Autodesk Inventor part; units mm, degrees
ref_plane "YZ Plane" through (0, 0, 0) normal (1, 0, 0) x (0, 1, 0)
ref_plane "XZ Plane" through (0, 0, 0) normal (0, 1, 0) x (-1, 0, 0)
ref_plane "XY Plane" through (0, 0, 0) normal (0, 0, 1) x (1, 0, 0)
ref_plane "РабПлоскость1" through (0, 0, 0) normal (0, 0, 1) x (1, 0, 0)
sketch "Эскиз1" plane through (0, 0, 0) normal (0, 0, 1) x (1, 0, 0)
  circle A0 centre (-0.0013, 107.169) radius 13.15
  circle A1 centre (-0.0025, 107.6908) radius 11.9
  point P0 (0, 0)
extrude "Выдавливание1" add sketch "Эскиз1" against normal blind 10 contours A0 | A1
sketch "Эскиз2" plane through (-0.0013, 107.169, 0) normal (0, 0, 1) x (1, 0, 0)
  circle A0 centre (0, 0) radius 15.5
  point P0 (0.0013, -107.169)
  dimension "d2" = 31
extrude "Выдавливание2" add sketch "Эскиз2" along normal blind 5.2
sketch "Эскиз3" plane through (-0.0013, 107.169, 5.2) normal (0, 0, 1) x (1, 0, 0)
  circle A0 centre (0, 0) radius 11.9
  point P0 (0.0013, -107.169)
  dimension "d5" = 23.8
extrude "Выдавливание3" add sketch "Эскиз3" along normal blind 20
sketch "Эскиз4" plane through (-0.0013, 107.169, 25.2) normal (0, 0, 1) x (1, 0, 0)
  circle A0 centre (0, 0) radius 6.5
  point P0 (0.0013, -107.169)
  dimension "d8" = 13
extrude "Выдавливание4" cut sketch "Эскиз4" against normal up to next
properties part number "Ось"
Part model, mm, in its own coordinate system. A direction names the side the tool comes from. Give positions to 0.01 mm unless a question says otherwise; leave off trailing zeros. Order: outer loops, then holes, each group sorted by start corner. A loop starts at its lowest first (then second) coordinate and runs counter-clockwise, first axis right, second up. Notation, with made-up numbers: (76, 11) - (107, 11) arc R23 ccw to (107, 41) - close; hole circle Ø11 at (52, 40). An arc over 180 degrees is marked (long way). One line per question, with ' | ' between items.
1. Pull direction X, two halves, no side cores. Call faces 4 (the face through (5, 96, 5.2)), 5 (the face through (-1.41, 100.824, 7.846)), 6 (the face through (-2.85, 94.33, -4.93)): +X half, -X half, draft (parallel to the pull), parting line (faces both ways), or undercut.
Filled in:
face 4: draft | face 5: undercut | face 6: parting line
2. Drill centre lines: probe 1 along X at (y, z) = (107, -2); probe 2 along Z at (x, y) = (-10, 97); probe 3 along X at (y, z) = (102, -6). Where is each one in solid material? Low to high.
Filled in:
probe 1: -13.15 to -6.5, 6.5 to 13.15 | probe 2: 0 to 5.2 | probe 3: -12.09 to -3.94, 3.94 to 12.09
3. Band-saw the part on B-B on y = 103. List the corners of the cut face in (x, z).
Filled in:
outline: (-14.93, 0) - (-12.47, 0) - (-12.47, -10) - (-4.99, -10) - (-4.99, 25.2) - (-11.15, 25.2) - (-11.15, 5.2) - (-14.93, 5.2) - close; (4.99, -10) - (12.47, -10) - (12.47, 0) - (14.93, 0) - (14.93, 5.2) - (11.14, 5.2) - (11.14, 25.2) - (4.99, 25.2) - close
4. Which spindle directions (+Z, -Z, +X, -X, +Y, -Y) get a long thin tool onto all of the face, cutting with end or side? Do faces 1 (the face through (-2.581, 118.786, 15.06)), 2 (the face through (-7, 95.8, 0)), 3 (the face through (-6, 104, -10)). Say none if no direction does.
Filled in:
face 1: +Z | face 2: -Z | face 3: -Z, +X, -X, +Y, -Y
5. Band-saw the part on D-D on x = -11. List the corners of the cut face in (y, z), then the cut area to 3 significant figures.
Filled in:
outline: (96.25, 0) - (99.96, 0) - (99.96, -10) - (114.38, -10) - (114.38, 0) - (118.09, 0) - (118.09, 5.2) - (111.71, 5.2) - (111.71, 25.2) - (102.63, 25.2) - (102.63, 5.2) - (96.25, 5.2) - close | area: 439 mm²
6. Band-saw the part on C-C on y = 116.5. List the corners of the cut face in (x, z), then the cut area to 3 significant figures.
Filled in:
outline: (-12.38, 0) - (-9.27, 0) - (-9.27, -10) - (9.26, -10) - (9.26, 0) - (12.38, 0) - (12.38, 5.2) - (7.38, 5.2) - (7.38, 25.2) - (-7.39, 25.2) - (-7.39, 5.2) - (-12.38, 5.2) - close | area: 609 mm²
7. Drop flat-ended pins along their axis: P1, Ø10, axis at x = -10, z = 3, coming from the +Y side; P2, Ø1, axis at x = 11, z = -1, coming from the +Y side; P3, Ø8, axis at x = 0, y = 107.17, coming from the +Z side; P4, Ø2, axis at y = 110.5, z = 1, coming from the +X side. Give the stop position or say it passes through.
Filled in:
P1: y = 121.84 | P2: y = 115.08 | P3: through | P4: x = 15.32
8. Band-saw the part on A-A on x = 0. List the corners of the cut face in (y, z), then the cut area to 3 significant figures.
Filled in:
outline: (91.67, 0) - (94.02, 0) - (94.02, -10) - (100.67, -10) - (100.67, 25.2) - (95.27, 25.2) - (95.27, 5.2) - (91.67, 5.2) - close; (113.67, -10) - (120.32, -10) - (120.32, 0) - (122.67, 0) - (122.67, 5.2) - (119.07, 5.2) - (119.07, 25.2) - (113.67, 25.2) - close | area: 443 mm²
